Autodesk Inventor part; units mm, degrees
ref_plane "XZ Plane" through (0, 0, 0) normal (0, 1, 0) x (-1, 0, 0)
sketch "Эскиз1" plane through (0, 0, 0) normal (0, 1, 0) x (-1, 0, 0)
  line L0 (-11.45, -11.25) -> (11.45, -11.25)
  line L1 (11.45, -11.25) -> (11.45, 11.25)
  line L2 (11.45, 11.25) -> (-11.45, 11.25)
  line L3 (-11.45, 11.25) -> (-11.45, -11.25)
  line L4 (-11.45, -11.25) -> (11.45, 11.25) construction
  line L5 (11.45, -11.25) -> (-11.45, 11.25) construction
  point P0 (0, 0)
  dimension "d0" = 22.5
  dimension "d1" = 22.9
extrude "Выдавливание1" add sketch "Эскиз1" along normal blind 2
sketch "Эскиз2" plane through (0, 2, 0) normal (0, 1, 0) x (1, 0, 0)
  line L0 (-11.45, 11.25) -> (-11.45, -11.25)
  line L1 (-11.45, -11.25) -> (0, 0)
  circle A0 centre (-7.9663, -7.8272) radius 2
  line L2 (15.4928, 0) -> (-16.8416, 0)
  line L3 (0, -16.9938) -> (0, 16.458)
  circle A1 centre (-7.9663, 7.8272) radius 2
  circle A2 centre (7.9663, -7.8272) radius 2
  circle A3 centre (7.9663, 7.8272) radius 2
  dimension "d8" = 4
extrude "Выдавливание2" cut sketch "Эскиз2" against normal blind 2 contours A0 L1 | L1 A0 | A1 | A2 | A3
fillet "Сопряжение1" radius 2 4 edges at (-11.45, 1, 11.25) (11.45, 1, 11.25) (11.45, 1, -11.25) (-11.45, 1, -11.25)
properties part number "энкодер"
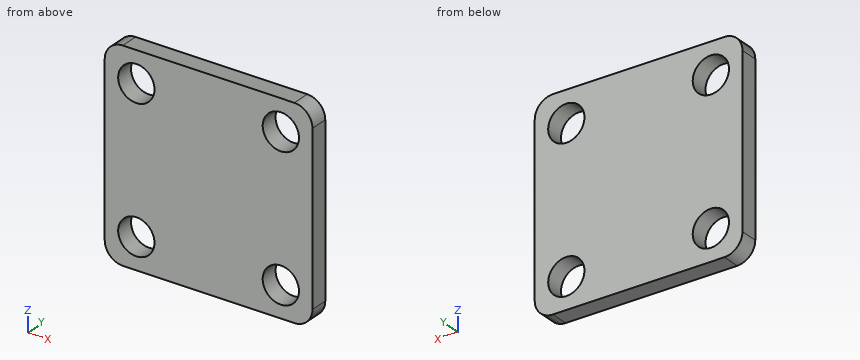
Can you work these out from the model? Positions are in its coordinate system, mm. Round coordinates to 2 decimals unless told otherwise and drop trailing zeros. Loops run counter-clockwise (first coordinate to the right, second up) from the corner with the lowest first, then second, coordinate; pieces in that order, holes last. Notation, with made-up numbers: (54, 19.25) - (87, 19.25) arc R13 ccw to (87, 24.25) - close; hole circle Ø1 at (45, -5.75). An arc over 180 degrees is marked (long way). Answer in a Markdown table with one row per item. Add a question column.
Q1. For pin 1 Ø2.5 at (x, z) = (7.97, 7.83) entering from +Y, with a flat end and sliding along its axis, tell me the tip position at first contact or that it passes through.
Q2. I want a section at A-A on x = 6.5. List the corners of the cut face in (y, z) for me.
Q3. I need wall thicknesses on L1, parallel to Z at x = -9.75, y = 1.3; L2, parallel to Z at x = 7.5, y = 1.5; L3, parallel to X at y = 0.85, z = -6.75. Which ranges of each line are inside material? Lowest first, please.
Q4. I want a section at B-B on y = 0.35. List the corners of the cut face in (x, z) for me.
A:
| question | item | result |
|---|---|---|
| 1 | pin 1 | through |
| 2 | outline | (0, -11.25) - (2, -11.25) - (2, -9.19) - (0, -9.19) - close; (0, -6.47) - (2, -6.47) - (2, 6.47) - (0, 6.47) - close; (0, 9.19) - (2, 9.19) - (2, 11.25) - (0, 11.25) - close |
| 3 | L1 | -11.23 to -8.73, -6.92 to 6.92, 8.73 to 11.23 |
| 3 | L2 | -11.25 to -9.77, -5.88 to 5.88, 9.77 to 11.25 |
| 3 | L3 | -11.45 to -9.65, -6.28 to 6.28, 9.65 to 11.45 |
| 4 | outline | (-11.45, -9.25) arc R2 ccw to (-9.45, -11.25) - (9.45, -11.25) arc R2 ccw to (11.45, -9.25) - (11.45, 9.25) arc R2 ccw to (9.45, 11.25) - (-9.45, 11.25) arc R2 ccw to (-11.45, 9.25) - close; hole circle Ø4 at (-7.97, -7.83); hole circle Ø4 at (-7.97, 7.83); hole circle Ø4 at (7.97, -7.83); hole circle Ø4 at (7.97, 7.83) |
